CAD build for the part. Positions are in the model's coordinates, mm. A direction names the side the tool comes from. Give positions to 0.01 mm unless a question says otherwise; leave off trailing zeros. Order: outer loops, then holes, each group sorted by start corner. A loop starts at its lowest first (then second) coordinate and runs counter-clockwise, first axis right, second up.
Item 1: Two-plate mould, pull along Z, no slides. Class faces 4 (the cylindrical face through (64.46, 7.64, -6.72)), 5 (the flat face through (16, 13, 0)), 6 (the cylindrical face through (-5.91, 7.64, -5.77)), 7 (the cylindrical face through (29, 8, 20)): released by +Z, released by -Z, zero draft, split by the parting line, or undercut.
Item 2: Band-saw the part on D-D on x = 48. Give the cut face in (y, z).
Item 3: Flat gauge pins, fed straight in: P1, Ø1.5, axis at x = -2.5, y = 5.5, coming from the -Z side; P2, Ø1.5, axis at x = 39, y = 5.5, coming from the +Z side; P3, Ø8, axis at y = 5, z = -19, coming from the +X side. Where does each tip first touch, or does it go through?
Item 4: Band-saw the part on A-A on y = 9.75. Give the cut face in (x, z), plus the area to 3 significant figures.
Item 5: Which spindle directions (+Z, -Z, +X, -X, +Y, -Y) get a long thin tool onto all of the face, cutting with end or side? Do faces 1 (the cylindrical face through (-25.2, 7.42, 24.34)), 2 (the flat face through (-63.5, 17.5, 5.9)), 3 (the cylindrical face through (-7.51, 7.42, -24.69)). Say none if no direction does.
Item 6: Band-saw the part on C-C on x = -55. Give the cut face in (y, z).
Item 7: Band-saw the part on B-B on z = -6. Count the separate pieces of the cut face and the enclosed holes in it, plus the area to 3 significant figures.
Item 8: Wall check: L1, parallel to X at y = 10.25, z = 0; L2, parallel to X at y = 12.5, z = 10; L3, parallel to Z at x = -75, y = 7. Give the ranges that are in metal, low to high.
Autodesk Fusion 360 part; units mm, degrees
sketch "Sketch1" plane through (0, 0, 0) normal (0, 1, 0) x (1, 0, 0)
  line L0 (75, -25) -> (-75, -25)
  line L1 (-75, -25) -> (-75, 25)
  line L2 (-75, 25) -> (75, 25)
  line L3 (75, 25) -> (75, -25)
  line L4 (75, -25) -> (-75, 25) construction
  line L5 (-75, -25) -> (75, 25) construction
  circle A0 centre (-75, 0) radius 25
  circle A1 centre (75, 0) radius 25
  dimension "d1" = 150
  dimension "d2" = 50
extrude "Extrude1" add sketch "Sketch1" along normal blind 15
sketch "Sketch2" plane through (0, 15, 0) normal (0, 1, 0) x (-1, 0, 0)
  arc A0 (75, -25) -> (75, 25) centre (75, 0) ccw
  line L0 (75, 25) -> (-75, 25)
  arc A1 (-75, 25) -> (-75, -25) centre (-75, 0) ccw
  line L1 (-75, -25) -> (75, -25)
  circle A2 centre (75, 0) radius 25
  circle A3 centre (-75, 0) radius 25
  circle A4 centre (17, 0) radius 22.5
  dimension "d5" = 50
  dimension "d6" = 50
  dimension "d7" = 45
  dimension "d8" = 25
  dimension "d9" = 45
  dimension "d10" = 58
extrude "Extrude2" add sketch "Sketch2" along normal blind 2.5 contours A0 A2 | A1 A3 | A4
sketch "Sketch3" plane through (0, 0, 0) normal (0, -1, 0) x (1, 0, 0)
  arc A0 (-75, 25) -> (-75, -25) centre (-75, 0) ccw
  line L0 (-75, -25) -> (75, -25)
  arc A1 (75, -25) -> (75, 25) centre (75, 0) ccw
  line L1 (75, 25) -> (-75, 25)
  circle A2 centre (-75, 0) radius 25
  circle A3 centre (-17, 0) radius 22.5
  circle A4 centre (75, 0) radius 25
  dimension "d13" = 45
  dimension "d14" = 58
  dimension "d15" = 45
  dimension "d16" = 25
  dimension "d17" = 50
  dimension "d18" = 50
extrude "Extrude3" add sketch "Sketch3" along normal blind 2.5 contours A0 A2 | A1 A4 | A3
sketch "Sketch4" plane through (0, -2.5, 0) normal (0, -1, 0) x (1, 0, 0)
  circle A0 centre (-75, 0) radius 25
  line L0 (-75, 0) -> (-75, 15.3312)
  line L1 (-17, 0) -> (-17, 15)
  line L2 (75, 0) -> (75, 15)
  dimension "d21" = 15
  dimension "d22" = 15
  dimension "d29" = 58
  dimension "d30" = 92
hole "Hole1" at (-75, -2.5, 0) at (-17, -2.5, 0) at (75, -2.5, 0) direction (0, 1, 0) diameter 25 depth 20 tip angle 118
sketch "Sketch5" plane through (0, 15, 0) normal (0, 1, 0) x (-1, 0, 0)
  arc A0 (-75, -25) -> (-75, 25) centre (-75, 0) ccw
  line L0 (-75, -25) -> (75, -25)
  arc A1 (75, 25) -> (75, -25) centre (75, 0) ccw
  line L1 (75, 25) -> (-75, 25)
  circle A2 centre (17, 0) radius 22.5
  line L2 (17, 0) -> (17, -25)
  line L3 (17, -25) -> (7, -25)
  line L4 (17, 0) -> (17, 25)
  line L5 (17, 25) -> (7, 25)
  line L6 (-75, -25) -> (-65, -25)
  line L7 (-75, 25) -> (-65, 25)
  line L8 (7, 25) -> (-29, 25)
  line L9 (-29, 25) -> (-29, -20)
  line L10 (-29, 25) -> (-29, 20)
  arc A3 (7, -25) -> (-65, -25) centre (-29, -152.1) ccw
  arc A4 (-65, 25) -> (7, 25) centre (-29, 152.1) ccw
  line L11 (75, 25) -> (65, 25)
  line L12 (75, -25) -> (65, -25)
  line L13 (17, -25) -> (27, -25)
  line L14 (17, 25) -> (27, 25)
  line L15 (65, 25) -> (46, 25)
  line L16 (46, 25) -> (46, 20)
  line L17 (46, 20) -> (46, -20)
  arc A5 (65, -25) -> (27, -25) centre (46, -58.6) ccw
  arc A6 (27, 25) -> (65, 25) centre (46, 58.6) ccw
  dimension "d31" = 10
  dimension "d32" = 10
  dimension "d33" = 36
  dimension "d34" = 45
  dimension "d35" = 19
  dimension "d36" = 40
  dimension "d37" = 29
  dimension "d38" = 132.1
  dimension "d39" = 132.1
  dimension "d40" = 10
  dimension "d41" = 38.6
  dimension "d42" = 38.6
  dimension "d43" = 10
  dimension "d44" = 10
  dimension "d45" = 10
extrude "Extrude4" cut sketch "Sketch5" against normal blind 15 contours L0 A3 | L1 L9 L10 A4 | L1 L8 L9 L10 A4 | L0 A5 | L1 L16 A6 | L1 L15 L16 A6
fillet "Fillet1" radius 45 8 edges at (-65, 7.5, -25) (-27, 7.5, -25) (-7, 7.5, -25) (65, 7.5, -25) (-65, 7.5, 25) (-27, 7.5, 25) (-7, 7.5, 25) (65, 7.5, 25)
extrude "Extrude5" cut 1 faces at (21.1667, 0, 0) along direction (0, 1, 0) blind 2
extrude "Extrude6" cut 1 faces at (21.1667, 15, 0) along direction (0, -1, 0) blind 2
equation "d33 = ( 72 / 2 ) * 1 mm"
equation "d35 = ( 38 / 2 ) * 1 mm"
The answers:
1. face 4: undercut
1. face 5: zero draft
1. face 6: undercut
1. face 7: released by +Z
2. outline: (2, -21.37) - (13, -21.37) - (13, 21.37) - (2, 21.37) - close
3. P1: stops at z = -23.98
3. P2: stops at z = 20.44
3. P3: stops at x = 95
4. outline: (-75, -25) - (-74.48, -25) arc R45 ccw to (-59.15, -22.31) arc R38.6 cw to (-32.85, -22.31) arc R45 ccw to (-17.52, -25) - (-12.79, -25) arc R45 ccw to (-2.17, -23.73) arc R132.1 cw to (60.17, -23.73) arc R45 ccw to (70.79, -25) - (75, -25) arc R25 ccw to (75, 25) - (70.79, 25) arc R45 ccw to (60.17, 23.73) arc R132.1 cw to (-2.17, 23.73) arc R45 ccw to (-12.79, 25) - (-17.52, 25) arc R45 ccw to (-32.85, 22.31) arc R38.6 cw to (-59.15, 22.31) arc R45 ccw to (-74.48, 25) - (-75, 25) arc R25 ccw to start; hole circle Ø25 at (-75, 0); hole circle Ø25 at (-17, 0); hole circle Ø25 at (75, 0)
4. area: 7,230 mm2
5. face 1: +Z, +Y, -Y
5. face 2: +Z, -Z, +X, -X, +Y
5. face 3: -Z, +Y, -Y
6. outline: (-2.5, -15) - (2, -15) - (2, -21.06) - (13, -21.06) - (13, -15) - (17.5, -15) - (17.5, 15) - (13, 15) - (13, 21.06) - (2, 21.06) - (2, 15) - (-2.5, 15) - close
7. separate pieces: 4
7. enclosed holes: 0
7. area: 2,130 mm2
8. L1: x = -100 to -87.5, -62.5 to -29.5, -4.5 to 62.5, 87.5 to 100
8. L2: x = -97.91 to -82.5, -67.5 to -24.5, -9.5 to 67.5, 82.5 to 97.91
8. L3: z = -25 to -12.5, 12.5 to 25
